Check sheet for the modelled part. Datum: model origin and axes. Units: mm. A direction names the side the tool comes from. Round coordinates to 2 decimals unless told otherwise and drop trailing zeros. Loops run counter-clockwise (first coordinate to the right, second up) from the corner with the lowest first, then second, coordinate; pieces in that order, holes last. Notation, with made-up numbers: (47.25, 55.5) - (72.25, 55.5) arc R6 ccw to (72.25, 65.5) - close; hole circle Ø6 at (-17.75, -4.5). An arc over 180 degrees is marked (long way). Put each result on its own line as item: value.
```python
from build123d import *

# Parameters (mm, degrees)
F0_W      = 17
F0_H      = 3
F1_DEPTH  = 14
F0_H_2    = 147
F1_FACE_W = 17
F1_FACE_H = 3
F2_DEPTH  = 3
F3_R      = 1.5
F4_DEPTH  = 25
F5_R      = 2.75
F6_DEPTH  = 25
F7_R      = 1.5


with BuildPart() as f1:
    # F0 (on Top) → F1 (new body)
    with BuildSketch(Plane.XY):
        with Locations((0, -73.5)):
            Rectangle(F0_W, F0_H)
    extrude(amount=F1_DEPTH)

    # F0 (on Top) + F1_face (on face) → F2 (join)
    with BuildSketch(Plane.XY):
        with Locations((0, 1.5)):
            Rectangle(F0_W, F0_H_2)
    with BuildSketch(Plane(origin=(0, -73.5, 0), x_dir=(1, 0, 0), z_dir=(0, 0, -1))):
        Rectangle(F1_FACE_W, F1_FACE_H)
    extrude(amount=-F2_DEPTH, dir=(0, 0, 1))

    # F3 (on face) → F4 (cut)
    with BuildSketch(Plane(origin=(0, -72, 0), x_dir=(-1, 0, 0), z_dir=(0, 1, 0))):
        with Locations((0, 7)):
            Circle(F3_R)
    extrude(amount=-F4_DEPTH, mode=Mode.SUBTRACT)

    # F5 (on face) → F6 (cut)
    with BuildSketch(Plane.XY):
        with Locations((0, -1)):
            Circle(F5_R)
        with Locations((0, 25)):
            Circle(F5_R)
    extrude(amount=-F6_DEPTH, mode=Mode.SUBTRACT)

    # F7
    f7_edges = [f1.edges().sort_by_distance(p)[0] for p in [
        (0, -75, -3),
        (0, -72, 0),
    ]]
    fillet(f7_edges, radius=F7_R)


solid = f1.part
```
Item 1: Section check A-A on y = 25. Enter the section's corners in (x, z), then the cut area to 3 significant figures.
Filled sheet:
outline: (-8.5, -3) - (-2.75, -3) - (-2.75, 0) - (-8.5, 0) - close; (2.75, -3) - (8.5, -3) - (8.5, 0) - (2.75, 0) - close
area: 34.5 mm²
Item 2: Tool access check on faces 1 (the cylindrical face through (-2.182, -2.673, -1.479)), 2 (the flat face through (0, -72, 9)). Record the directions out of +Z, -Z, +X, -X, +Y, -Y that give a thin tool (end or side, any length) a straight path to the whole face; none if there is none.
Filled sheet:
face 1: +Z, -Z
face 2: +Z, +X, -X, +Y
Item 3: Thickness scan on line 1 (Y direction, x = 0, z = -1.1); line 2 (Z direction, x = 0, y = -73.3); line 3 (Z direction, x = -3, y = 44.5). Record the ranges inside material, lowest first. Write a range as from..to.
Filled sheet:
line 1: -75..-3.75, 1.75..22.25, 27.75..75
line 2: -3..5.5, 8.5..14
line 3: -3..0
Item 4: Section check C-C on x = 0. Enter the section's corners in (y, z), then the cut area to 3 significant figures.
Filled sheet:
outline: (-75, -1.5) arc R1.5 ccw to (-73.5, -3) - (-3.75, -3) - (-3.75, 0) - (-70.5, 0) arc R1.5 cw to (-72, 1.5) - (-72, 5.5) - (-75, 5.5) - close; (-75, 8.5) - (-72, 8.5) - (-72, 14) - (-75, 14) - close; (1.75, -3) - (22.25, -3) - (22.25, 0) - (1.75, 0) - close; (27.75, -3) - (75, -3) - (75, 0) - (27.75, 0) - close
area: 450 mm²
Item 5: Release check for a two-part mould opening along X. For faces 3 (the cylindrical face through (0.325, -73.479, 5.536)), 4 (the flat face through (0, -75, 5)), 5 (the flat face through (-8.5, -11, -1)) record: +X half, -X half, draft (parallel to the pull), parting line (faces both ways), or undercut.
Filled sheet:
face 3: undercut
face 4: draft
face 5: -X half
Item 6: Go/stop test with flat-tipped pins: pin 1 (6.5 mm diameter, centred on x = 0, y = -1, fed in from +Z); pin 2 (10 mm diameter, centred on x = 2, z = 8.5, fed in from +Y). Record where each tip stops, or that it passes through.
Filled sheet:
pin 1: z = 0
pin 2: y = -72
Item 7: Section check B-B on z = 7. Enter the section's corners in (x, y), then the cut area to 3 significant figures.
Filled sheet:
outline: (-8.5, -75) - (-1.5, -75) - (-1.5, -72) - (-8.5, -72) - close; (1.5, -75) - (8.5, -75) - (8.5, -72) - (1.5, -72) - close
area: 42.0 mm²
Item 8: Section check D-D on x = -6. Enter the section's corners in (y, z).
Filled sheet:
outline: (-75, -1.5) arc R1.5 ccw to (-73.5, -3) - (75, -3) - (75, 0) - (-70.5, 0) arc R1.5 cw to (-72, 1.5) - (-72, 14) - (-75, 14) - close
